from build123d import *

# Parameters (mm, degrees)
SKETCH1_W                       = 25.4
SKETCH1_H                       = 25.4
SKETCH1_W_2                     = 19.05
SKETCH1_H_2                     = 19.05
EXTRUDE_THIN1_DEPTH             = 501.65
F_3_16_0_1875_DIAMETER_HOLE1_D  = 4.7625
F_1_4_0_25_DIAMETER_HOLE1_D     = 6.35
F_1_4_0_25_DIAMETER_HOLE1_DEPTH = 25.4
F_1_4_0_25_DIAMETER_HOLE1_TIP   = 1.907732465
F_1_4_CLEARANCE_HOLE1_D         = 6.7564
F_1_4_CLEARANCE_HOLE1_DEPTH     = 38.1
F_1_4_CLEARANCE_HOLE1_TIP       = 2.029827343


with BuildPart() as part:
    # Sketch1 → Extrude-Thin1 (new body)
    with BuildSketch(Plane.XY):
        Rectangle(SKETCH1_W, SKETCH1_H)
        Rectangle(SKETCH1_W_2, SKETCH1_H_2, mode=Mode.SUBTRACT)
    extrude(amount=EXTRUDE_THIN1_DEPTH)

    # 3/16 (0.1875) Diameter Hole1 (through all)
    with Locations(Plane(origin=(0, 12.7, 495.3), x_dir=(0, 0, 1), z_dir=(0, 1, 0))):
        with Locations((0, 0), (-488.95, 0), (-463.55, 0), (-438.15, 0), (-25.4, 0), (-50.8, 0)):
            Hole(F_3_16_0_1875_DIAMETER_HOLE1_D / 2)

    # 1/4 (0.25) Diameter Hole1
    with Locations(Plane(origin=(0, 12.7, 0), x_dir=(1, 0, 0), z_dir=(0, 1, 0))):
        with Locations((0, -199.933463093), (0, -422.2), (0, -326.95), (0, -85.623539829)):
            Hole(F_1_4_0_25_DIAMETER_HOLE1_D / 2, depth=F_1_4_0_25_DIAMETER_HOLE1_DEPTH)
            with Locations((0, 0, -(F_1_4_0_25_DIAMETER_HOLE1_DEPTH + F_1_4_0_25_DIAMETER_HOLE1_TIP / 2))):  # 118° drill point
                Cone(0, F_1_4_0_25_DIAMETER_HOLE1_D / 2, F_1_4_0_25_DIAMETER_HOLE1_TIP, mode=Mode.SUBTRACT)

    # 1/4 Clearance Hole1
    with Locations(Plane(origin=(-381, 12.7, 250.825), x_dir=(1, 0, 0), z_dir=(0, 1, 0))):
        with Locations((381, 82.55), (381, 98.425), (381, 114.3), (381, -146.05), (381, -130.175), (381, -114.3), (-381, -146.05), (-381, -130.175), (-381, -114.3), (-381, 82.55), (-381, 98.425), (-381, 114.3)):
            Hole(F_1_4_CLEARANCE_HOLE1_D / 2, depth=F_1_4_CLEARANCE_HOLE1_DEPTH)
            with Locations((0, 0, -(F_1_4_CLEARANCE_HOLE1_DEPTH + F_1_4_CLEARANCE_HOLE1_TIP / 2))):  # 118° drill point
                Cone(0, F_1_4_CLEARANCE_HOLE1_D / 2, F_1_4_CLEARANCE_HOLE1_TIP, mode=Mode.SUBTRACT)


solid = part.part
Could you check a few things on this model? Use its own coordinates, in mm. A direction names the side the tool comes from. Round coordinates to 2 decimals unless told otherwise and drop trailing zeros. Write each loop counter-clockwise with the first axis right and the second up, starting at its lowest first coordinate (ties: lowest second). Pieces come first, ordered by that corner, then holes. Notation, with made-up numbers: (88, -4) - (106, -4) arc R31 ccw to (106, 35) - close; hole circle Ø3 at (-20.75, 11.25). An arc over 180 degrees is marked (long way). Put each result on its own line as item: value. Start each with the question number.
(1) Thinking about a two-plate mould opening in Y: for faces 3 (the flat face through (-12.7, 0, 247)), 4 (the flat face through (0, -9.525, 247)), 5 (the flat face through (0, 12.7, 247)), which applies, released by +Y, released by -Y, zero draft, split by the parting line, or undercut?
(2) I want a section at A-A, the plane y = 1. Please give me the cut outline in (x, z) (3 decimals).
(3) Will this pin go through, and if not, where does the flat tip stop? pin 1 (3 mm diameter, centred on x = 0, z = 57.15, fed in from +Y).
(4) I need wall thicknesses on probe 1 along X at (y, z) = (3, 100) (3 decimals); probe 2 along X at (y, z) = (11.1, 326.95) (3 decimals). Which ranges of each line are inside material? Lowest first, please.
(5) For faces 1 (the flat face through (11, 0, 501.65)), 2 (the flat face through (-9.525, 0, 247)), which set-ups out of +Z, -Z, +X, -X, +Y, -Y let a thin tool reach every point of the face, with its end or its side?
(6) I want a section at B-B, the plane z = 345.5. Please give me the cut outline in (x, y) (3 decimals).
Here are the results:
1. face 3: zero draft
1. face 4: undercut
1. face 5: released by +Y
2. outline: (-12.7, 0) - (-9.525, 0) - (-9.525, 501.65) - (-12.7, 501.65) - close; (9.525, 0) - (12.7, 0) - (12.7, 501.65) - (9.525, 501.65) - close
3. pin 1: passes through
4. probe 1: x = -12.7 to -9.525, 9.525 to 12.7
4. probe 2: x = -12.7 to -3.175, 3.175 to 12.7
5. face 1: +Z, +X, -X, +Y, -Y
5. face 2: +Z, -Z
6. outline: (-12.7, -12.7) - (12.7, -12.7) - (12.7, 12.7) - (-12.7, 12.7) - close; hole (-9.525, -9.525) - (9.525, -9.525) - (9.525, 9.525) - (-9.525, 9.525) - close
